Verification items for the finished model (mm, model axes). A direction names the side the tool comes from. Round coordinates to 2 decimals unless told otherwise and drop trailing zeros. Write each loop counter-clockwise with the first axis right and the second up, starting at its lowest first coordinate (ties: lowest second). Pieces come first, ordered by that corner, then holes. Notation, with made-up numbers: M 40.25,30 L 58.25,30 A19 cw 58.25,50 Z; hole C 1.5,19.25 d9. An arc over 180 degrees is marked long. Write each question's results on one line, items separated by ' | '.
from build123d import *

# Parameters (mm, degrees)
CROQUIS1_W                = 5
CROQUIS1_H                = 2
SALIENTE_EXTRUIR1_DEPTH   = 36
CROQUIS1_W_2              = 2
CROQUIS1_H_2              = 5
SALIENTE_EXTRUIR1_2_DEPTH = 36
SALIENTE_EXTRUIR1_3_DEPTH = 36
SALIENTE_EXTRUIR1_4_DEPTH = 36
SALIENTE_EXTRUIR1_5_DEPTH = 36
CROQUIS2_W                = 79
CROQUIS2_H                = 39
SALIENTE_EXTRUIR2_DEPTH   = 2
CORTAR_EXTRUIR1_DEPTH     = 36
CROQUIS4_W                = 5
CROQUIS4_H                = 2
SALIENTE_EXTRUIR3_DEPTH   = 36
CROQUIS5_W                = 10
CROQUIS5_H                = 2
SALIENTE_EXTRUIR4_DEPTH   = 12
NERVIO1_REACH             = 88.442
CROQUIS8_WALL_W           = 190.62700295
CROQUIS8_WALL_H           = 1
NERVIO2_REACH             = 80.309
CROQUIS9_WALL_W           = 174.36001667
CROQUIS9_WALL_H           = 1
NERVIO3_REACH             = 88.442
CROQUIS10_WALL_W          = 190.62700295
CROQUIS10_WALL_H          = 1
NERVIO4_REACH             = 80.309
CROQUIS11_WALL_W          = 174.36001667
CROQUIS11_WALL_H          = 1
CROQUIS12_R               = 2
CORTAR_EXTRUIR2_DEPTH     = 64.217877218


with BuildPart() as part:
    # Croquis1 → Saliente-Extruir1 (new body)
    with BuildSketch(Plane(origin=(0, 0, 0), x_dir=(1, 0, 0), z_dir=(0, 1, 0))):
        with Locations((30, -18.5)):
            Rectangle(CROQUIS1_W, CROQUIS1_H)
    extrude(amount=SALIENTE_EXTRUIR1_DEPTH)



with BuildPart() as body_2:
    # Croquis1 → Saliente-Extruir1 2 (new body)
    with BuildSketch(Plane(origin=(0, 0, 0), x_dir=(1, 0, 0), z_dir=(0, 1, 0))):
        with Locations((38.5, -10)):
            Rectangle(CROQUIS1_W_2, CROQUIS1_H_2)
    extrude(amount=SALIENTE_EXTRUIR1_2_DEPTH)


with BuildPart() as body_3:
    # Croquis1 → Saliente-Extruir1 3 (new body)
    with BuildSketch(Plane(origin=(0, 0, 0), x_dir=(1, 0, 0), z_dir=(0, 1, 0))):
        Polygon((39.5, 19.5), (27.5, 19.5), (27.5, 17.5), (37.5, 17.5), (37.5, 7.5), (39.5, 7.5), align=None)
    extrude(amount=SALIENTE_EXTRUIR1_3_DEPTH)


with BuildPart() as body_4:
    # Croquis1 → Saliente-Extruir1 4 (new body)
    with BuildSketch(Plane(origin=(0, 0, 0), x_dir=(1, 0, 0), z_dir=(0, 1, 0))):
        Polygon((-39.5, 7.5), (-39.5, 19.5), (-27.5, 19.5), (-27.5, 17.5), (-37.5, 17.5), (-37.5, 7.5), align=None)
    extrude(amount=SALIENTE_EXTRUIR1_4_DEPTH)


with BuildPart() as body_5:
    # Croquis1 → Saliente-Extruir1 5 (new body)
    with BuildSketch(Plane(origin=(0, 0, 0), x_dir=(1, 0, 0), z_dir=(0, 1, 0))):
        Polygon((-39.5, -7.5), (-39.5, -19.5), (-27.5, -19.5), (-27.5, -17.5), (-37.5, -17.5), (-37.5, -7.5), align=None)
    extrude(amount=SALIENTE_EXTRUIR1_5_DEPTH)


with BuildPart() as part_1:
    add(part.part)

    add(body_2.part)  # Saliente-Extruir2 merges body 2

    add(body_3.part)  # Saliente-Extruir2 merges body 3

    add(body_4.part)  # Saliente-Extruir2 merges body 4

    add(body_5.part)  # Saliente-Extruir2 merges body 5
    # Croquis2 → Saliente-Extruir2 (add)
    with BuildSketch(Plane.XZ):
        Rectangle(CROQUIS2_W, CROQUIS2_H)
    extrude(amount=SALIENTE_EXTRUIR2_DEPTH)

    # Croquis3 → Cortar-Extruir1 (cut)
    with BuildSketch(Plane(origin=(0, 36, 0), x_dir=(1, 0, 0), z_dir=(0, 1, 0))):
        Polygon((-32.5, -17.5), (-32.5, -19.5), (-39.5, -19.5), (-39.5, -12.5), (-37.5, -12.5), (-37.5, -17.5), align=None)
    extrude(amount=-CORTAR_EXTRUIR1_DEPTH, mode=Mode.SUBTRACT)

    # Croquis4 → Saliente-Extruir3 (add)
    with BuildSketch(Plane(origin=(0, 0, 0), x_dir=(1, 0, 0), z_dir=(0, 1, 0))):
        with Locations((-25, -18.5)):
            Rectangle(CROQUIS4_W, CROQUIS4_H)
        with Locations((25, -18.5)):
            Rectangle(CROQUIS4_W, CROQUIS4_H)
    extrude(amount=SALIENTE_EXTRUIR3_DEPTH)

    # Croquis5 → Saliente-Extruir4 (add)
    with BuildSketch(Plane.XY.offset(19.5)):
        with Locations((-27.5, 35)):
            Rectangle(CROQUIS5_W, CROQUIS5_H)
        with Locations((27.5, 35)):
            Rectangle(CROQUIS5_W, CROQUIS5_H)
    extrude(amount=SALIENTE_EXTRUIR4_DEPTH)

    # Croquis8 wall → Nervio1 (add, up to next)
    with BuildSketch(Plane(origin=(-32.5, 28.90512554, 25.5), x_dir=(0, -0.647270304875, -0.762260554159), z_dir=(0, -0.762260554159, 0.647270304875)), mode=Mode.PRIVATE) as nervio1_sk1:
        with Locations((0, 0.5)):
            Rectangle(CROQUIS8_WALL_W, CROQUIS8_WALL_H)
    nervio1_tool1 = extrude(nervio1_sk1.sketch, amount=-NERVIO1_REACH, mode=Mode.PRIVATE) - part_1.part
    add(nervio1_tool1.solids().sort_by_distance((-32.5, 28.90512554, 25.5))[0])

    # Croquis9 wall → Nervio2 (add, up to next)
    with BuildSketch(Plane(origin=(-22.5, 28.90512554, 25.5), x_dir=(0, -0.647270304875, -0.762260554159), z_dir=(0, 0.762260554159, -0.647270304875)), mode=Mode.PRIVATE) as nervio2_sk1:
        with Locations((0, 0.5)):
            Rectangle(CROQUIS9_WALL_W, CROQUIS9_WALL_H)
    nervio2_tool1 = extrude(nervio2_sk1.sketch, amount=NERVIO2_REACH, mode=Mode.PRIVATE) - part_1.part
    add(nervio2_tool1.solids().sort_by_distance((-22.5, 28.90512554, 25.5))[0])

    # Croquis10 wall → Nervio3 (add, up to next)
    with BuildSketch(Plane(origin=(32.5, 28.90512554, 25.5), x_dir=(0, -0.647270304875, -0.762260554159), z_dir=(0, 0.762260554159, -0.647270304875)), mode=Mode.PRIVATE) as nervio3_sk1:
        with Locations((0, 0.5)):
            Rectangle(CROQUIS10_WALL_W, CROQUIS10_WALL_H)
    nervio3_tool1 = extrude(nervio3_sk1.sketch, amount=NERVIO3_REACH, mode=Mode.PRIVATE) - part_1.part
    add(nervio3_tool1.solids().sort_by_distance((32.5, 28.90512554, 25.5))[0])

    # Croquis11 wall → Nervio4 (add, up to next)
    with BuildSketch(Plane(origin=(22.5, 28.90512554, 25.5), x_dir=(0, 0.647270304875, 0.762260554159), z_dir=(0, 0.762260554159, -0.647270304875)), mode=Mode.PRIVATE) as nervio4_sk1:
        with Locations((0, 0.5)):
            Rectangle(CROQUIS11_WALL_W, CROQUIS11_WALL_H)
    nervio4_tool1 = extrude(nervio4_sk1.sketch, amount=NERVIO4_REACH, mode=Mode.PRIVATE) - part_1.part
    add(nervio4_tool1.solids().sort_by_distance((22.5, 28.90512554, 25.5))[0])

    # Croquis12 → Cortar-Extruir2 (cut, through all)
    with BuildSketch(Plane(origin=(0, 36, 0), x_dir=(1, 0, 0), z_dir=(0, 1, 0))):
        with Locations(Location((27.5, -24.5, 0), (0, 0, 270))):
            Circle(CROQUIS12_R)
        with Locations(Location((-27.5, -24.5, 0), (0, 0, 270))):
            Circle(CROQUIS12_R)
    extrude(amount=-CORTAR_EXTRUIR2_DEPTH, mode=Mode.SUBTRACT)


solid = part_1.part
1) Depth check by flat-ended pin: P1, Ø15.5, axis at y = 23.5, z = 21, coming from the -X side; P2, Ø2, axis at x = 39, y = 19, coming from the +Z side; P3, Ø12, axis at x = -22, z = -8, coming from the +Y side. Enter the tip coordinate at first touch or a pass-through.
Calculated:
P1: stops at x = -32.5 | P2: stops at z = 12.5 | P3: stops at y = 0
2) Access from +Z, -Z, +X, -X, +Y, -Y to the whole of each face (thin tool, end or side, straight path). Record for faces 4 (the flat face through (31.5, 31, 24)), 5 (the flat face through (32.5, 26, 21)), 6 (the flat face through (27, 18, 17.5)), 7 (the flat face through (37.5, 18, 10)).
Calculated:
face 4: +Z, -Y | face 5: +Z, +X, +Y | face 6: +X, -X, +Y | face 7: +Z, +Y
3) Sectioned sample at B-B, the plane z = 8.5. Record the cut outline in (x, y), and give its area (3 significant figures).
Calculated:
outline: M -39.5,-2 L 39.5,-2 L 39.5,36 L 37.5,36 L 37.5,0 L -37.5,0 L -37.5,36 L -39.5,36 Z | area: 302 mm²
4) Sectioned sample at A-A, the plane y = 19.5. Record the cut outline in (x, z).
Calculated:
outline: M -39.5,-19.5 L -27.5,-19.5 L -27.5,-17.5 L -37.5,-17.5 L -37.5,-7.5 L -39.5,-7.5 Z; M -39.5,7.5 L -37.5,7.5 L -37.5,12.5 L -39.5,12.5 Z; M -32.5,17.5 L -22.5,17.5 L -22.5,19.5 L -32.5,19.5 Z; M 22.5,17.5 L 32.5,17.5 L 32.5,19.5 L 22.5,19.5 Z; M 27.5,-19.5 L 39.5,-19.5 L 39.5,-7.5 L 37.5,-7.5 L 37.5,-17.5 L 27.5,-17.5 Z; M 37.5,7.5 L 39.5,7.5 L 39.5,12.5 L 37.5,12.5 Z
5) Sectioned sample at D-D, the plane z = 21. Record the cut outline in (x, y).
Calculated:
outline: M -32.5,25.08 L -31.5,25.08 L -31.5,34 L -23.5,34 L -23.5,25.08 L -22.5,25.08 L -22.5,36 L -32.5,36 Z; M 22.5,25.08 L 23.5,25.08 L 23.5,34 L 31.5,34 L 31.5,25.08 L 32.5,25.08 L 32.5,36 L 22.5,36 Z
6) Material ranges on line 1 (X direction, y = 34.5, z = 24.5); line 2 (X direction, y = 6.5, z = -8); line 3 (X direction, y = 29, z = 20), recorded low to high. Write a range as [from, to].
Calculated:
line 1: x = [-32.5, -29.5], [-25.5, -22.5], [22.5, 25.5], [29.5, 32.5] | line 2: x = [-39.5, -37.5], [37.5, 39.5] | line 3: x = [-32.5, -31.5], [-23.5, -22.5], [22.5, 23.5], [31.5, 32.5]
7) Sectioned sample at C-C, the plane x = -34. Record the cut outline in (y, z).
Calculated:
outline: M -2,-19.5 L 36,-19.5 L 36,-17.5 L 0,-17.5 L 0,19.5 L -2,19.5 Z
8) Draft check along Z on faces 1 (the flat face through (38, 36, 10)), 2 (the flat face through (-6, -1, 19.5)), 3 (the cylindrical face through (25.548, 35.014, 24.066)). Enter one of: pulls with the +Z half, pulls with the -Z half, needs draft (parallel to the pull), parting line crosses it, or undercut.
Calculated:
face 1: needs draft | face 2: pulls with the +Z half | face 3: undercut
